Geometry: final body of the model. Coordinates: model frame, mm. A direction names the side the tool comes from. Give positions to 0.01 mm unless a question says otherwise; leave off trailing zeros. Write each loop counter-clockwise with the first axis right and the second up, starting at its lowest first coordinate (ties: lowest second). Pieces come first, ordered by that corner, then holes. Notation, with made-up numbers: (46, -20.75) - (87, -20.75) arc R16 ccw to (87, 0.25) - close; hole circle Ø6 at (73, 46.5). An arc over 180 degrees is marked (long way). Use CSV: the item, a comma, the result in double quotes. Start each with the question number.
(1) Reachability of faces 1 (the flat face through (92, 614, 0)), 2 (the flat face through (165, 554, 0)), 3 (the flat face through (13, 0, 22)) from +Z, -Z, +X, -X, +Y, -Y: full face, straight path, thin tool, end or side. Return the list, or none.
(2) Section C-C on y = 221. Output: boundary loops of the cut face in (x, z).
(3) Section A-A on x = 83. Output: boundary loops of the cut face in (y, z).
(4) Line query: probe 1 along Y at (x, z) = (101.5, -1.5); probe 2 along Y at (x, z) = (106.5, 2.5); probe 3 along Y at (x, z) = (20, -15.5). Output: solid intervals per line, ascending. Write a range as [from, to].
(5) First-contact query: pin 1 Ø8 at (x, y) = (17.5, -93.5) entering from -Z; pin 2 Ø3 at (x, z) = (134.5, -2.5) entering from +Y; pin 3 Ø0.5 at (x, z) = (28, -5) entering from +Y. Flat tips, straight axial feed; report the tip coordinate or a pass-through.
(6) Section B-B on y = -229.5. Output: boundary loops of the cut face in (x, z).
(7) Draft query along X for faces 4 (the flat face through (92, 642, 0)), 5 (the cylindrical face through (23.846, -19.72, 7.509)), 6 (the flat face through (96.05, 524.82, 0.14)), 7 (the flat face through (65, 630, 10)). Return one class per face: released by +X, released by -X, zero draft, split by the parting line, or undercut.
from build123d import *

# Parameters (mm, degrees)
F0_R      = 29
F1_DEPTH  = 750
F2_R      = 25
F3_DEPTH  = 40
F4_R      = 29
F4_R_2    = 25
F5_DEPTH  = 44
F6_R      = 22
F7_DEPTH  = 196
F8_R      = 43
F8_R_2    = 22
F9_DEPTH  = 75
F10_SIZE2 = 25
F10_SIZE  = 6
F11_W     = 6
F11_H     = 12
F12_DEPTH = 10


# Not quite as in the source:
# - a feature names something its author has since deleted; it is built from what else it names


with BuildPart() as f1:
    # F0 (on Front) → F1 (new body)
    with BuildSketch(Plane.XZ):
        Circle(F0_R)
    extrude(amount=-F1_DEPTH)

    # F2 (on Front) → F3 (join)
    with BuildSketch(Plane.XZ):
        Circle(F2_R)
    extrude(amount=F3_DEPTH)

    # F4 (on face) → F5 (join)
    with BuildSketch(Plane.XZ.offset(40)):
        Circle(F4_R)
        Circle(F4_R_2, mode=Mode.SUBTRACT)
        Circle(F4_R_2)
    extrude(amount=F5_DEPTH)

    # F6 (on face) → F7 (join)
    with BuildSketch(Plane.XZ.offset(84)):
        Circle(F6_R)
    extrude(amount=F7_DEPTH)

    # F8 (on face) → F9 (join)
    with BuildSketch(Plane.XZ.offset(280)):
        Circle(F8_R)
        Circle(F8_R_2, mode=Mode.SUBTRACT)
        Circle(F8_R_2)
    extrude(amount=F9_DEPTH)

    # F10
    f10_edges = [f1.edges().sort_by_distance(p)[0] for p in [
        (-29, 750, 0),
    ]]
    f10_side = f1.faces().sort_by_distance((-29, 375, 0))[0]
    chamfer(f10_edges, length=F10_SIZE, length2=F10_SIZE2, reference=f10_side)

    # F11 (on Top) → F12 (join, symmetric)
    with BuildSketch(Plane.XY):
        Polygon((164.9999544621, 717.9999580383), (28.9999544621, 743.9999580383), (28.9999544621, 717.9999580383), align=None)
        Polygon((28.9999544621, 717.9999580383), (28.9999544621, 743.9999580383), (3.9999544621, 743.9999580383), (3.9999544621, 511.9999580383), (28.9999544621, 511.9999580383), (28.9999544621, 537.9999580383), align=None)
        Polygon((164.9999544621, 717.9999580383), (28.9999544621, 717.9999580383), (28.9999544621, 537.9999580383), (164.9999544621, 537.9999580383), (164.9999544621, 557.9999580383), (92.9999544621, 557.9999580383), (92.9999544621, 591.9999580383), (66.9999544621, 591.9999580383), (66.9999544621, 599.9999580383), (66.9999544621, 627.9999580383), (66.9999544621, 655.9999580383), (92.9999544621, 655.9999580383), (92.9999544621, 663.9999580383), (92.9999544621, 697.9999580383), (164.9999544621, 697.9999580383), align=None)
        Polygon((164.9999544621, 537.9999580383), (28.9999544621, 537.9999580383), (28.9999544621, 511.9999580383), align=None)
        Polygon((164.9999544621, 685.9999580383), (164.9999544621, 697.9999580383), (92.9999544621, 697.9999580383), align=None)
        Polygon((116.9999544621, 663.9999580383), (92.9999544621, 697.9999580383), (92.9999544621, 663.9999580383), align=None)
        Polygon((92.9999544621, 557.9999580383), (164.9999544621, 557.9999580383), (164.9999544621, 569.9999580383), align=None)
        Polygon((116.9999544621, 663.9999580383), (92.9999544621, 663.9999580383), (92.9999544621, 655.9999580383), (116.9999544621, 655.9999580383), (132.9999544621, 655.9999580383), (138.9999544621, 655.9999580383), (150.9999544621, 655.9999580383), (150.9999544621, 663.9999580383), (138.9999544621, 663.9999580383), (132.9999544621, 663.9999580383), align=None)
        Polygon((132.9999544621, 675.9999580383), (116.9999544621, 663.9999580383), (132.9999544621, 663.9999580383), align=None)
        Polygon((92.9999544621, 591.9999580383), (92.9999544621, 557.9999580383), (116.9999544621, 591.9999580383), align=None)
        Polygon((116.9999544621, 655.9999580383), (92.9999544621, 655.9999580383), (66.9999544621, 655.9999580383), (66.9999544621, 627.9999580383), align=None)
        with Locations((135.9999544621, 669.9999580383)):
            Rectangle(F11_W, F11_H)
        Polygon((66.9999544621, 591.9999580383), (92.9999544621, 591.9999580383), (116.9999544621, 591.9999580383), (132.9999544621, 591.9999580383), (138.9999544621, 591.9999580383), (150.9999544621, 591.9999580383), (150.9999544621, 599.9999580383), (138.9999544621, 599.9999580383), (132.9999544621, 599.9999580383), (116.9999544621, 599.9999580383), (66.9999544621, 599.9999580383), align=None)
        Polygon((132.9999544621, 591.9999580383), (116.9999544621, 591.9999580383), (132.9999544621, 579.9999580383), align=None)
        Polygon((132.9999544621, 655.9999580383), (116.9999544621, 655.9999580383), (132.9999544621, 643.9999580383), align=None)
        Polygon((138.9999544621, 675.9999580383), (138.9999544621, 663.9999580383), (150.9999544621, 663.9999580383), align=None)
        with Locations((135.9999544621, 585.9999580383)):
            Rectangle(F11_W, F11_H)
        with Locations((135.9999544621, 649.9999580383)):
            Rectangle(F11_W, F11_H)
        Polygon((116.9999544621, 599.9999580383), (66.9999544621, 627.9999580383), (66.9999544621, 599.9999580383), align=None)
        Polygon((150.9999544621, 591.9999580383), (138.9999544621, 591.9999580383), (138.9999544621, 579.9999580383), align=None)
        Polygon((150.9999544621, 655.9999580383), (138.9999544621, 655.9999580383), (138.9999544621, 643.9999580383), align=None)
        Polygon((132.9999544621, 611.9999580383), (116.9999544621, 599.9999580383), (132.9999544621, 599.9999580383), align=None)
        with Locations((135.9999544621, 605.9999580383)):
            Rectangle(F11_W, F11_H)
        Polygon((138.9999544621, 599.9999580383), (150.9999544621, 599.9999580383), (138.9999544621, 611.9999580383), align=None)
    extrude(amount=F12_DEPTH, both=True)


solid = f1.part
Check values:
1,face 1,"+Z, -Z"
1,face 2,"+Z, -Z, +X, +Y, -Y"
1,face 3,"none"
2,outline,"circle Ø58 at (0, 0)"
3,outline,"(522.32, -10) - (619.04, -10) - (619.04, 10) - (522.32, 10) - close; (636.96, -10) - (733.68, -10) - (733.68, 10) - (636.96, 10) - close"
4,probe 1,"y = [525.86, 559.42], [570.04, 608.68], [647.32, 685.96], [696.58, 730.14]"
4,probe 2,"y = [526.82, 560.25], [577.13, 605.88], [650.12, 678.87], [695.75, 729.18]"
4,probe 3,"y = [-355, -280], [-84, -40], [0, 744.89]"
5,pin 1,"stops at z = -17.37"
5,pin 2,"stops at y = 724.12"
5,pin 3,"stops at y = 744.19"
6,outline,"circle Ø44 at (0, 0)"
7,face 4,"undercut"
7,face 5,"split by the parting line"
7,face 6,"released by +X"
7,face 7,"zero draft"
